Verification items for the finished model (mm, model axes). Face numbers are marked on the shaded views. A direction names the side the tool comes from. Coordinates: 2 decimals unless noted, no trailing zeros. Write each loop counter-clockwise with the first axis right and the second up, starting at its lowest first coordinate (ties: lowest second). Pieces come first, ordered by that corner, then holes.
```python
from build123d import *

# Parameters (mm, degrees)
SKETCH1_W                 = 43
SKETCH1_H                 = 43
BOSS_EXTRUDE1_DEPTH       = 5
FILLET1_R                 = 3
F_4_0MM_DOWEL_HOLE1_D     = 4
F_4_0MM_DOWEL_HOLE1_DEPTH = 10
F_4_0MM_DOWEL_HOLE1_TIP   = 1.201721238
SKETCH5_R                 = 5.5
CUT_EXTRUDE1_DEPTH        = 5
SKETCH6_W                 = 5
SKETCH6_H                 = 43
BOSS_EXTRUDE2_DEPTH       = 38
BOSS_EXTRUDE2_DEPTH_BACK  = 5
CUT_EXTRUDE4_START        = -5
SKETCH11_R                = 12.25
CUT_EXTRUDE4_DEPTH        = 2
SKETCH12_W                = 43
SKETCH12_H                = 5
BOSS_EXTRUDE3_DEPTH       = 40
SKETCH13_R                = 3.571875
CUT_EXTRUDE5_DEPTH        = 10
SKETCH15_R                = 6.75
CUT_EXTRUDE6_DEPTH        = 38
BOSS_EXTRUDE4_DEPTH       = 2.5
LPATTERN1_COUNT           = 3
LPATTERN1_PITCH           = 20.25
BOSS_EXTRUDE5_DEPTH       = 5.141078
BOSS_EXTRUDE5_DEPTH_BACK  = 7.641078
BOSS_EXTRUDE6_DEPTH       = 5


with BuildPart() as part:
    # Sketch1 → Boss-Extrude1 (new body)
    with BuildSketch(Plane(origin=(0, 0, 0), x_dir=(1, 0, 0), z_dir=(0, 1, 0))):
        with Locations((21.5, -22.047500095)):
            Rectangle(SKETCH1_W, SKETCH1_H)
    extrude(amount=BOSS_EXTRUDE1_DEPTH)

    # Fillet1
    fillet1_edges = [part.edges().sort_by_distance(p)[0] for p in [
        (0, 2.5, 0.547500095),
        (0, 2.5, 43.547500095),
    ]]
    fillet(fillet1_edges, radius=FILLET1_R)

    # Ø4.0mm Dowel Hole1
    with Locations(Plane(origin=(0, 5, 0), x_dir=(1, 0, 0), z_dir=(0, 1, 0))):
        with Locations((6, -6.547500095), (37, -6.547500095), (37, -37.547500095), (6, -37.547500095)):
            Hole(F_4_0MM_DOWEL_HOLE1_D / 2, depth=F_4_0MM_DOWEL_HOLE1_DEPTH)
            with Locations((0, 0, -(F_4_0MM_DOWEL_HOLE1_DEPTH + F_4_0MM_DOWEL_HOLE1_TIP / 2))):  # 118° drill point
                Cone(0, F_4_0MM_DOWEL_HOLE1_D / 2, F_4_0MM_DOWEL_HOLE1_TIP, mode=Mode.SUBTRACT)

    # Sketch5 → Cut-Extrude1 (cut)
    with BuildSketch(Plane(origin=(0, 5, 0), x_dir=(1, 0, 0), z_dir=(0, 1, 0))):
        with Locations((21.939339828, -22.486839923)):
            Circle(SKETCH5_R)
    extrude(amount=-CUT_EXTRUDE1_DEPTH, mode=Mode.SUBTRACT)

    # Sketch6 → Boss-Extrude2 (add, two sides)
    with BuildSketch(Plane(origin=(0, 5, 0), x_dir=(1, 0, 0), z_dir=(0, 1, 0))) as boss_extrude2_sk:
        with Locations((45.5, -22.047500095)):
            Rectangle(SKETCH6_W, SKETCH6_H)
    extrude(amount=BOSS_EXTRUDE2_DEPTH)
    extrude(boss_extrude2_sk.sketch, amount=-BOSS_EXTRUDE2_DEPTH_BACK)

    # Sketch11 → Cut-Extrude4 (cut)
    with BuildSketch(Plane.XZ.offset(CUT_EXTRUDE4_START)):
        with Locations((21.939339828, 22.486839923)):
            Circle(SKETCH11_R)
    extrude(amount=CUT_EXTRUDE4_DEPTH, mode=Mode.SUBTRACT)

    # Sketch12 → Boss-Extrude3 (add)
    with BuildSketch(Plane(origin=(48, 0, 0), x_dir=(0, 0, -1), z_dir=(1, 0, 0))):
        with Locations((-22.047500095, 40.5)):
            Rectangle(SKETCH12_W, SKETCH12_H)
    extrude(amount=BOSS_EXTRUDE3_DEPTH)

    # Sketch13 → Cut-Extrude5 (cut)
    with BuildSketch(Plane(origin=(0, 38, 0), x_dir=(-1, 0, 0), z_dir=(0, -1, 0))):
        with Locations((-50.4, -9.347500095)):
            Circle(SKETCH13_R)
        with Locations((-50.4, -34.747500095)):
            Circle(SKETCH13_R)
    extrude(amount=-CUT_EXTRUDE5_DEPTH, mode=Mode.SUBTRACT)

    # Sketch15 → Cut-Extrude6 (cut)
    with BuildSketch(Plane.XZ.offset(-38)):
        with Locations((50.4, 9.347500095)):
            Circle(SKETCH15_R)
        with Locations((50.4, 34.747500095)):
            Circle(SKETCH15_R)
    extrude(amount=CUT_EXTRUDE6_DEPTH, mode=Mode.SUBTRACT)

    # Sketch16 → Boss-Extrude4 (add)
    with BuildSketch(Plane(origin=(0, 0, 0.547500095), x_dir=(-1, 0, 0), z_dir=(0, 0, -1))):
        Polygon((-48, 9.800798491), (-74.261330934, 38), (-48, 38), align=None)
    boss_extrude4 = extrude(amount=-BOSS_EXTRUDE4_DEPTH)

    # LPattern1: Boss-Extrude4 ×3
    with Locations(*[(0, 0, i * LPATTERN1_PITCH) for i in range(1, LPATTERN1_COUNT)]):
        add(boss_extrude4)

    # Sketch18 → Boss-Extrude5 (add, two sides)
    with BuildSketch(Plane(origin=(0, 0, 20.797500095), x_dir=(-1, 0, 0), z_dir=(0, 0, -1))) as boss_extrude5_sk:
        Polygon((-48, 38), (-48, 9.800798491), (-74.261330934, 38), align=None)
    extrude(amount=BOSS_EXTRUDE5_DEPTH)
    extrude(boss_extrude5_sk.sketch, amount=-BOSS_EXTRUDE5_DEPTH_BACK)

    # Sketch19 → Boss-Extrude6 (add)
    with BuildSketch(Plane(origin=(0, 0, 0), x_dir=(-1, 0, 0), z_dir=(0, -1, 0))):
        Polygon((-15, 5.802499905), (-36, 5.802499905), (-36, -0.547500095), (-41, -0.547500095), (-41, 10.802499905), (-10, 10.802499905), (-10, -0.547500095), (-15, -0.547500095), align=None)
    extrude(amount=-BOSS_EXTRUDE6_DEPTH)


solid = part.part
```
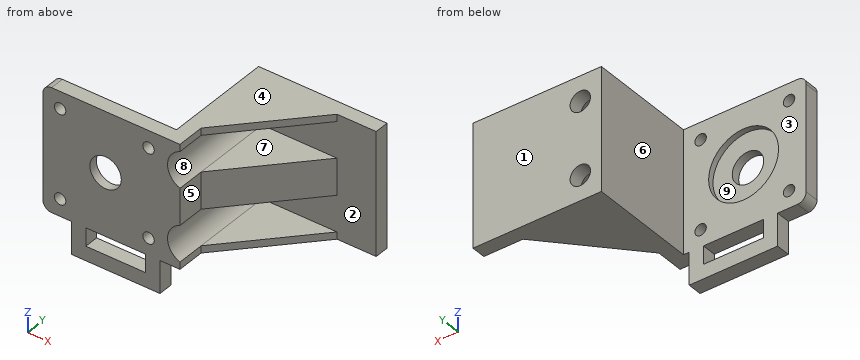
1. Sectioned sample at C-C, the plane z = 32.5. Record the boundary of the cut face in (x, y).
2. Gauge pin test, flat ends, axial feed: P1, Ø13, axis at x = 63.5, y = 20.5, coming from the -Z side; P2, Ø3, axis at y = 3, z = 19, coming from the +X side; P3, Ø6, axis at y = 27.5, z = 5.5, coming from the +X side; P4, Ø6.5, axis at x = 50.4, z = 34.75, coming from the -Y side. Record the tip position at first contact, or that the pin passes through.
3. Sectioned sample at D-D, the plane x = 37. Record the boundary of the cut face in (y, z).
4. Tool access check on the marked faces 1, 2, 3, 4 and 5. Record the directions out of +Z, -Z, +X, -X, +Y, -Y that give a thin tool (end or side, any length) a straight path to the whole face; none if there is none.
5. Sectioned sample at B-B, the plane y = 6.5. Record the boundary of the cut face in (x, z).
6. Sectioned sample at A-A, the plane x = 6. Record the boundary of the cut face in (y, z).
7. Draft check along X on the marked faces 6, 7, 8 and 9. Enter one of: pulls with the +X half, pulls with the -X half, needs draft (parallel to the pull), parting line crosses it, or undercut.
8. Material ranges on L1, parallel to Z at x = 53, y = 28.5; L2, parallel to Z at x = 6, y = 1.05; L3, parallel to Y at x = 12, z = 9, recorded low to high.
Outcome:
1. outline: (0, 0) - (44.04, 0) - (44.04, 38) - (47.62, 38) - (47.62, 43) - (43, 43) - (43, 5) - (29, 5) - (29, 3) - (14.88, 3) - (14.88, 5) - (0, 5) - close; (53.18, 38) - (88, 38) - (88, 43) - (53.18, 43) - close
2. P1: stops at z = 0.55
2. P2: stops at x = 48
2. P3: stops at x = 66.09
2. P4: passes through
3. outline: (0, -10.8) - (5, -10.8) - (5, 4.55) - (0, 4.55) - close; (0, 8.55) - (5, 8.55) - (5, 35.55) - (0, 35.55) - close; (0, 39.55) - (5, 39.55) - (5, 43.55) - (0, 43.55) - close
4. face 1: +Z, -Z, +X, -X, +Y
4. face 2: +X, -Y
4. face 3: +Z, -Z, -X, +Y
4. face 4: +Z, +X, -X, +Y, -Y
4. face 5: +Z, -Z, +X, -Y
5. outline: (43, 0.55) - (48, 0.55) - (48, 3.04) arc R6.75 cw to (48, 15.66) - (48, 28.44) arc R6.75 cw to (48, 41.06) - (48, 43.55) - (43, 43.55) - close
6. outline: (0, 0.55) - (5, 0.55) - (5, 4.55) - (0, 4.55) - close; (0, 8.55) - (5, 8.55) - (5, 35.55) - (0, 35.55) - close; (0, 39.55) - (5, 39.55) - (5, 43.55) - (0, 43.55) - close
7. face 6: pulls with the -X half
7. face 7: needs draft
7. face 8: pulls with the +X half
7. face 9: undercut
8. L1: z = 0.55 to 3.05, 15.66 to 28.44, 41.05 to 43.55
8. L2: z = 0.55 to 4.55, 8.55 to 35.55, 39.55 to 43.55
8. L3: y = 0 to 5
